Geometry: final body of the model. Coordinates: model frame, mm. A direction names the side the tool comes from. Give positions to 0.01 mm unless a question says otherwise; leave off trailing zeros. Loops run counter-clockwise (first coordinate to the right, second up) from the corner with the lowest first, then second, coordinate; pieces in that order, holes last. Notation, with made-up numbers: (59, -7) - (90, -7) arc R22 ccw to (90, 14) - close; hole circle Ø8 at (86, 47). An arc over 180 degrees is marked (long way). Answer in a Markdown table with one row per item.
from build123d import *

# Parameters (mm, degrees)
SKETCH_1_W          = 37.2
SKETCH_1_H          = 22.3
SKETCH_1_R          = 0.75
EXTRUDE_1_DEPTH     = 5
SKETCH_1_3_W        = 37.2
SKETCH_1_3_H        = 22.3
SKETCH_1_3_R        = 0.75
CUT_EXTRUDE_2_DEPTH = 3.5
EXTRUDE_3_DEPTH     = 9
SKETCH_4_W          = 10.4
SKETCH_4_H          = 7.5
EXTRUDE_4_DEPTH     = 3.5


with BuildPart() as part:
    # 草圖1 → 填料-伸長1 (new body)
    with BuildSketch(Plane.XY):
        with Locations((63.739258578, 17.893460251)):
            Rectangle(SKETCH_1_W, SKETCH_1_H)
        with Locations((78.839258578, 8.593460251)):
            Circle(SKETCH_1_R, mode=Mode.SUBTRACT)
        with Locations((52.239258578, 27.193460251)):
            Circle(SKETCH_1_R, mode=Mode.SUBTRACT)
        with Locations((52.239258578, 8.593460251)):
            Circle(SKETCH_1_R, mode=Mode.SUBTRACT)
    extrude(amount=EXTRUDE_1_DEPTH)

    # 草圖1<3> → 除料-伸長2 (cut)
    with BuildSketch(Plane.XY):
        with Locations((63.739258578, 17.893460251)):
            Rectangle(SKETCH_1_3_W, SKETCH_1_3_H)
        with Locations((78.839258578, 8.593460251)):
            Circle(SKETCH_1_3_R, mode=Mode.SUBTRACT)
        with Locations((52.239258578, 27.193460251)):
            Circle(SKETCH_1_3_R, mode=Mode.SUBTRACT)
        with Locations((52.239258578, 8.593460251)):
            Circle(SKETCH_1_3_R, mode=Mode.SUBTRACT)
    extrude(amount=CUT_EXTRUDE_2_DEPTH, mode=Mode.SUBTRACT)

    # 草圖3 → 填料-伸長3 (add)
    with BuildSketch(Plane.XY.offset(5)):
        with BuildLine():
            Line((52.439258578, 14.193460251), (55.074078216, 14.193460251))
            ThreePointArc((55.074078216, 14.193460251), (76.639258578, 17.893460251), (55.074078216, 21.593460251))
            Line((55.074078216, 21.593460251), (52.439258578, 21.593460251))
            Line((52.439258578, 21.593460251), (52.439258578, 14.193460251))
        make_face()
    extrude(amount=EXTRUDE_3_DEPTH)

    # 草圖4 → 填料-伸長4 (add)
    with BuildSketch(Plane(origin=(0, 0, 3.5), x_dir=(-1, 0, 0), z_dir=(0, 0, -1))):
        with Locations((-66.639258578, 13.993460251)):
            Rectangle(SKETCH_4_W, SKETCH_4_H)
    extrude(amount=EXTRUDE_4_DEPTH)


solid = part.part
Q1. Draft query along X for faces 1 (the cylindrical face through (51.64, 26.74, 4.24)), 2 (the flat face through (45.139, 18, 4)), 3 (the flat face through (64, 18, 14)), 4 (the cylindrical face through (79.532, 8.306, 4.24)). Return one class per face: pulls with the +X half, pulls with the -X half, needs draft (parallel to the pull), parting line crosses it, or undercut.
Check values:
| item | result |
|---|---|
| face 1 | undercut |
| face 2 | pulls with the -X half |
| face 3 | needs draft |
| face 4 | undercut |
Q2. Cut plane A-A (x = 79). Output: boundary loops of the cut face in (y, z).
Check values:
| item | result |
|---|---|
| outline | (6.74, 3.5) - (7.86, 3.5) - (7.86, 5) - (6.74, 5) - close; (9.33, 3.5) - (29.04, 3.5) - (29.04, 5) - (9.33, 5) - close |
Q3. Cut plane D-D (x = 61). Output: boundary loops of the cut face in (y, z).
Check values:
| item | result |
|---|---|
| outline | (6.74, 3.5) - (29.04, 3.5) - (29.04, 5) - (28.02, 5) - (28.02, 14) - (7.76, 14) - (7.76, 5) - (6.74, 5) - close |
Q4. Reachability of faces 5 (the flat face through (71.839, 14, 2)), 6 (the flat face through (54, 14.193, 9)), 7 (the cylindrical face through (76.63, 17.46, 9.44)) from +Z, -Z, +X, -X, +Y, -Y: full face, straight path, thin tool, end or side. Return the list, or none.
Check values:
| item | result |
|---|---|
| face 5 | -Z, +X, +Y, -Y |
| face 6 | +Z, -X, -Y |
| face 7 | +Z |
Q5. Cut plane B-B (y = 17.25). Output: boundary loops of the cut face in (x, z).
Check values:
| item | result |
|---|---|
| outline | (45.14, 3.5) - (61.44, 3.5) - (61.44, 0) - (71.84, 0) - (71.84, 3.5) - (82.34, 3.5) - (82.34, 5) - (76.62, 5) - (76.62, 14) - (52.44, 14) - (52.44, 5) - (45.14, 5) - close |
Q6. Material intervals for line 1 along Z through (x, y) = (62.5, 27); line 2 along Z through (x, y) = (54.5, 23.25); line 3 along Y through (x, z) = (54, 10.75), sorted ascending.
Check values:
| item | result |
|---|---|
| line 1 | 3.5 to 14 |
| line 2 | 3.5 to 5 |
| line 3 | 14.19 to 21.59 |
Q7. First-contact query: pin 1 (2 mm diameter, centred on y = 22.5, z = 11, fed in from -X); pin 2 (1.3 mm diameter, centred on x = 53.5, z = 10.5, fed in from +Y); pin 3 (1.7 mm diameter, centred on x = 52.24, y = 27.19, fed in from -Z). Flat tips, straight axial feed; report the tip coordinate or a pass-through.
Check values:
| item | result |
|---|---|
| pin 1 | x = 52.44 |
| pin 2 | y = 21.59 |
| pin 3 | z = 3.5 |
Q8. Cut plane C-C (z = 1). Output: boundary loops of the cut face in (x, y).
Check values:
| item | result |
|---|---|
| outline | (61.44, 10.24) - (71.84, 10.24) - (71.84, 17.74) - (61.44, 17.74) - close |
